```python
from build123d import *

# Parameters (mm, degrees)
BOSS_EXTRUDE1_DEPTH = 10.16
CUT_EXTRUDE1_DEPTH  = 10
CHAMFER1_SIZE       = 0.25
CHAMFER1_SIZE2      = 1.27
SKETCH3_R           = 1.778
BOSS_EXTRUDE2_DEPTH = 0.152
SKETCH4_R           = 0.889
CUT_EXTRUDE2_DEPTH  = 5.08
BOSS_EXTRUDE3_START = 0.9525
BOSS_EXTRUDE3_DEPTH = 0.9525
BOSS_EXTRUDE4_START = 0.318
BOSS_EXTRUDE4_DEPTH = 0.318
BOSS_EXTRUDE5_START = 0.635
SKETCH9_R           = 1.143
BOSS_EXTRUDE5_DEPTH = 0.635
CUT_EXTRUDE3_REACH  = 18.592
SKETCH11_R          = 0.64
CUT_EXTRUDE4_DEPTH  = 6.7
SKETCH12_R          = 0.64
CUT_EXTRUDE6_DEPTH  = 4
CUT_EXTRUDE7_DEPTH  = 1.27
SKETCH15_R          = 0.125
CUT_EXTRUDE8_DEPTH  = 14.860565005


with BuildPart() as part:
    # Sketch1 → Boss-Extrude1 (new, symmetric)
    with BuildSketch(Plane(origin=(0, 0, 0), x_dir=(0, 0, -1), z_dir=(1, 0, 0))):
        Polygon((-9.94, -3.81), (2, -3.81), (2, 3.81), (-7.4, 3.81), (-7.4, 4.57), (-9.18, 4.57), (-9.94, 4.293), align=None)
    extrude(amount=BOSS_EXTRUDE1_DEPTH, both=True)

    # Sketch2 → Cut-Extrude1 (cut)
    with BuildSketch(Plane.XY.offset(9.94)):
        with BuildLine():
            Line((-0.809711007, -2.81), (0.809711007, -2.81))
            ThreePointArc((0.809711007, -2.81), (2.54, -3.3), (4.270288993, -2.81))
            Line((4.270288993, -2.81), (5.08, -2.81))
            Line((5.08, -2.81), (5.08, 2.81))
            Line((5.08, 2.81), (-5.08, 2.81))
            Line((-5.08, 2.81), (-5.08, -2.81))
            Line((-5.08, -2.81), (-4.270288993, -2.81))
            ThreePointArc((-4.270288993, -2.81), (-2.54, -3.3), (-0.809711007, -2.81))
        make_face()
    extrude(amount=-CUT_EXTRUDE1_DEPTH, mode=Mode.SUBTRACT)

    # Chamfer1
    chamfer1_edges = [part.edges().sort_by_distance(p)[0] for p in [
        (-5.08, 0, 9.94),
        (-4.675144497, -2.81, 9.94),
        (-2.54, -3.3, 9.94),
        (0, -2.81, 9.94),
        (2.54, -3.3, 9.94),
        (4.675144497, -2.81, 9.94),
        (5.08, 0, 9.94),
        (0, 2.81, 9.94),
    ]]
    chamfer1_side = [part.faces().sort_by_distance(p)[0] for p in [
        (-9.941239627, 0.2415, 9.94),
    ]]
    chamfer(chamfer1_edges, length=CHAMFER1_SIZE, length2=CHAMFER1_SIZE2, reference=chamfer1_side[0])

    # Sketch3 → Boss-Extrude2 (add)
    with BuildSketch(Plane.XY.offset(9.94)):
        with Locations(Location((-7.62, 0, 0), (0, 0, 180))):
            Circle(SKETCH3_R)
        with Locations(Location((7.76, 0, 0), (0, 0, 180))):
            Circle(SKETCH3_R)
    extrude(amount=BOSS_EXTRUDE2_DEPTH)

    # Sketch4 → Cut-Extrude2 (cut)
    with BuildSketch(Plane.XY.offset(10.092)):
        with Locations((-7.62, 0)):
            Circle(SKETCH4_R)
        with Locations((7.76, 0)):
            Circle(SKETCH4_R)
    extrude(amount=-CUT_EXTRUDE2_DEPTH, mode=Mode.SUBTRACT)

    # Sketch5 → Boss-Extrude3 (add)
    with BuildSketch(Plane.XY.offset(-0.06).offset(BOSS_EXTRUDE3_START)):
        with BuildLine():
            Line((-3.175, 2.81), (-3.175, 1.662881535))
            ThreePointArc((-3.175, 1.662881535), (-3.798650071, 1.258650071), (-4.202881535, 0.635))
            Line((-4.202881535, 0.635), (-5.08, 0.635))
            Line((-5.08, 0.635), (-5.08, -0.635))
            Line((-5.08, -0.635), (-4.202881535, -0.635))
            ThreePointArc((-4.202881535, -0.635), (-3.798650071, -1.258650071), (-3.175, -1.662881535))
            Line((-3.175, -1.662881535), (-3.175, -3.238329044))
            ThreePointArc((-3.175, -3.238329044), (-2.54, -3.3), (-1.905, -3.238329044))
            Line((-1.905, -3.238329044), (-1.905, -1.662881535))
            ThreePointArc((-1.905, -1.662881535), (-1.281349929, -1.258650071), (-0.877118465, -0.635))
            Line((-0.877118465, -0.635), (0, -0.635))
            Line((0, -0.635), (0, 0.635))
            Line((0, 0.635), (-0.877118465, 0.635))
            ThreePointArc((-0.877118465, 0.635), (-1.281349929, 1.258650071), (-1.905, 1.662881535))
            Line((-1.905, 1.662881535), (-1.905, 2.81))
            Line((-1.905, 2.81), (-3.175, 2.81))
        make_face()
    boss_extrude3 = extrude(amount=-BOSS_EXTRUDE3_DEPTH)

    # Mirror1: Boss-Extrude3 across plane
    add(boss_extrude3.mirror(Plane(origin=(0, 0, 0), x_dir=(0, 0, 1), z_dir=(1, 0, 0))))

    # Sketch8 → Boss-Extrude4 (add)
    with BuildSketch(Plane.XY.offset(0.8925).offset(BOSS_EXTRUDE4_START)):
        with BuildLine():
            Line((-4.202881535, 0.635), (-3.490380976, 0.635))
            ThreePointArc((-3.490380976, 0.635), (-2.54, 1.143), (-1.589619024, 0.635))
            Line((-1.589619024, 0.635), (-0.877118465, 0.635))
            Line((-0.877118465, 0.635), (0.877118465, 0.635))
            Line((0.877118465, 0.635), (1.589619024, 0.635))
            ThreePointArc((1.589619024, 0.635), (2.54, 1.143), (3.490380976, 0.635))
            Line((3.490380976, 0.635), (4.202881535, 0.635))
            Line((4.202881535, 0.635), (5.08, 0.635))
            Line((5.08, 0.635), (5.08, -0.635))
            Line((5.08, -0.635), (4.202881535, -0.635))
            ThreePointArc((4.202881535, -0.635), (3.798650071, -1.258650071), (3.175, -1.662881535))
            Line((3.175, -1.662881535), (3.175, -3.238329044))
            ThreePointArc((3.175, -3.238329044), (2.54, -3.3), (1.905, -3.238329044))
            Line((1.905, -3.238329044), (1.905, -1.662881535))
            ThreePointArc((1.905, -1.662881535), (1.281349929, -1.258650071), (0.877118465, -0.635))
            Line((0.877118465, -0.635), (-0.877118465, -0.635))
            ThreePointArc((-0.877118465, -0.635), (-1.281349929, -1.258650071), (-1.905, -1.662881535))
            Line((-1.905, -1.662881535), (-1.905, -3.238329044))
            ThreePointArc((-1.905, -3.238329044), (-2.54, -3.3), (-3.175, -3.238329044))
            Line((-3.175, -3.238329044), (-3.175, -1.662881535))
            ThreePointArc((-3.175, -1.662881535), (-3.798650071, -1.258650071), (-4.202881535, -0.635))
            Line((-4.202881535, -0.635), (-5.08, -0.635))
            Line((-5.08, -0.635), (-5.08, 0.635))
            Line((-5.08, 0.635), (-4.202881535, 0.635))
        make_face()
    extrude(amount=-BOSS_EXTRUDE4_DEPTH)

    # Sketch9 → Boss-Extrude5 (add)
    with BuildSketch(Plane.XY.offset(1.2105).offset(BOSS_EXTRUDE5_START)):
        with Locations(Location((-2.54, 0, 0), (0, 0, 146.251011404))):
            Circle(SKETCH9_R)
        with Locations(Location((2.54, 0, 0), (0, 0, 146.251011404))):
            Circle(SKETCH9_R)
    extrude(amount=-BOSS_EXTRUDE5_DEPTH)

    # Cut-Extrude3: up to this face of the body (flat: up to its plane)
    cut_extrude3_end = Plane(part.part.faces().sort_by_distance((0, 2.81, 4.414046423))[0])
    # Sketch10 → Cut-Extrude3 (cut, up to the picked face)
    with BuildSketch(Plane(origin=(0, 4.57, 0), x_dir=(1, 0, 0), z_dir=(0, 1, 0)), mode=Mode.PRIVATE) as cut_extrude3_sk1:
        Polygon((-2.04, -9.18), (-1.765, -9.94), (-3.315, -9.94), (-3.04, -9.18), align=None)
    cut_extrude3_tool1 = split(extrude(cut_extrude3_sk1.sketch, amount=-CUT_EXTRUDE3_REACH, mode=Mode.PRIVATE), bisect_by=cut_extrude3_end, keep=Keep.BOTH, mode=Mode.PRIVATE)
    # Sketch10 → Cut-Extrude3 (cut, up to the picked face)
    with BuildSketch(Plane(origin=(0, 4.57, 0), x_dir=(1, 0, 0), z_dir=(0, 1, 0)), mode=Mode.PRIVATE) as cut_extrude3_sk2:
        Polygon((-8.395, -9.94), (-8.12, -9.18), (-7.12, -9.18), (-6.845, -9.94), align=None)
    cut_extrude3_tool2 = split(extrude(cut_extrude3_sk2.sketch, amount=-CUT_EXTRUDE3_REACH, mode=Mode.PRIVATE), bisect_by=cut_extrude3_end, keep=Keep.BOTH, mode=Mode.PRIVATE)
    # Sketch10 → Cut-Extrude3 (cut, up to the picked face)
    with BuildSketch(Plane(origin=(0, 4.57, 0), x_dir=(1, 0, 0), z_dir=(0, 1, 0)), mode=Mode.PRIVATE) as cut_extrude3_sk3:
        Polygon((3.04, -9.18), (3.315, -9.94), (1.765, -9.94), (2.04, -9.18), align=None)
    cut_extrude3_tool3 = split(extrude(cut_extrude3_sk3.sketch, amount=-CUT_EXTRUDE3_REACH, mode=Mode.PRIVATE), bisect_by=cut_extrude3_end, keep=Keep.BOTH, mode=Mode.PRIVATE)
    # Sketch10 → Cut-Extrude3 (cut, up to the picked face)
    with BuildSketch(Plane(origin=(0, 4.57, 0), x_dir=(1, 0, 0), z_dir=(0, 1, 0)), mode=Mode.PRIVATE) as cut_extrude3_sk4:
        Polygon((8.12, -9.18), (8.395, -9.94), (6.845, -9.94), (7.12, -9.18), align=None)
    cut_extrude3_tool4 = split(extrude(cut_extrude3_sk4.sketch, amount=-CUT_EXTRUDE3_REACH, mode=Mode.PRIVATE), bisect_by=cut_extrude3_end, keep=Keep.BOTH, mode=Mode.PRIVATE)
    add(cut_extrude3_tool1.solids().sort_by(Axis((-2.54, 4.57, 9.58732), (0, -1, 0)))[0], mode=Mode.SUBTRACT)
    add(cut_extrude3_tool2.solids().sort_by(Axis((-7.62, 4.57, 9.58732), (0, -1, 0)))[0], mode=Mode.SUBTRACT)
    add(cut_extrude3_tool3.solids().sort_by(Axis((2.54, 4.57, 9.58732), (0, -1, 0)))[0], mode=Mode.SUBTRACT)
    add(cut_extrude3_tool4.solids().sort_by(Axis((7.62, 4.57, 9.58732), (0, -1, 0)))[0], mode=Mode.SUBTRACT)

    # Sketch11 → Cut-Extrude4 (cut)
    with BuildSketch(Plane.XZ.offset(3.81)):
        with Locations(Location((-7.62, 2, 0), (0, 0, 270))):
            Circle(SKETCH11_R)
        with Locations(Location((7.62, 2, 0), (0, 0, 270))):
            Circle(SKETCH11_R)
    extrude(amount=-CUT_EXTRUDE4_DEPTH, mode=Mode.SUBTRACT)

    # Sketch12 → Cut-Extrude6 (cut)
    with BuildSketch(Plane(origin=(0, 0, -2), x_dir=(-1, 0, 0), z_dir=(0, 0, -1))):
        with Locations((-7.76, 0)):
            Circle(SKETCH12_R)
        with Locations((7.62, 0)):
            Circle(SKETCH12_R)
    extrude(amount=-CUT_EXTRUDE6_DEPTH, mode=Mode.SUBTRACT)

    # Sketch13 → Cut-Extrude7 (cut, symmetric)
    with BuildSketch(Plane(origin=(2.54, 0, 0), x_dir=(0, 0, -1), z_dir=(1, 0, 0))):
        Polygon((2, -3.81), (2, 2.79), (1.49, 2.79), (1.49, 1.02), (0.73, 1.02), (0.73, -3.56), (-0.92, -3.56), (-1.17, -3.81), align=None)
    cut_extrude7 = extrude(amount=CUT_EXTRUDE7_DEPTH, both=True, mode=Mode.SUBTRACT)

    # Mirror2: Cut-Extrude7 across plane
    add(cut_extrude7.mirror(Plane(origin=(0, 0, 0), x_dir=(0, 0, 1), z_dir=(1, 0, 0))), mode=Mode.SUBTRACT)

    # Sketch15 → Cut-Extrude8 (cut, through all)
    with BuildSketch(Plane.XY.offset(1.8455)):
        with Locations((-2.54, 0)):
            Circle(SKETCH15_R)
        with Locations((2.54, 0)):
            Circle(SKETCH15_R)
    extrude(amount=-CUT_EXTRUDE8_DEPTH, mode=Mode.SUBTRACT)


solid = part.part
```
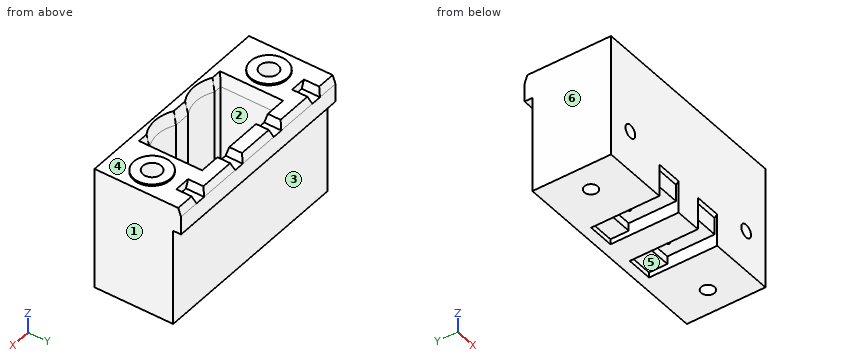
Part model, mm, in its own coordinate system. Face numbers are marked on the shaded views. A direction names the side the tool comes from. Round coordinates to 2 decimals unless told otherwise and drop trailing zeros. Loops run counter-clockwise (first coordinate to the right, second up) from the corner with the lowest first, then second, coordinate; pieces in that order, holes last.
1. Two-plate mould, pull along Y, no slides. Class the marked faces 1, 2 and 3: pulls with the +Y half, pulls with the -Y half, needs draft (parallel to the pull), parting line crosses it, or undercut.
Solutions:
face 1: needs draft
face 2: undercut
face 3: pulls with the +Y half
2. Slice it at D-D (z = 6.5). Give the cut face in (x, y), and give its area (3 significant figures).
Solutions:
outline: (-10.16, -3.81) - (10.16, -3.81) - (10.16, 3.81) - (-10.16, 3.81) - close; hole circle Ø1.78 at (-7.62, 0); hole (-5.08, -2.81) - (-4.27, -2.81) arc R3.3 ccw to (-0.81, -2.81) - (0.81, -2.81) arc R3.3 ccw to (4.27, -2.81) - (5.08, -2.81) - (5.08, 2.81) - (-5.08, 2.81) - close; hole circle Ø1.78 at (7.76, 0)
area: 90.5 mm2
3. 3-axis set-ups, long thin cutter, end or side, ignore diameter. For the marked faces 4, 5 and 6: which of +Z, -Z, +X, -X, +Y, -Y reach the whole face in a straight line?
Solutions:
face 4: +Z
face 5: -Z, -Y
face 6: +Z, -Z, -X, +Y, -Y
4. Slice it at A-A (y = 2.5). Give the cut face in (x, z) (1 decimal).
Solutions:
outline: (-10.2, -2) - (-3.8, -2) - (-3.8, -1.5) - (-1.3, -1.5) - (-1.3, -2) - (1.3, -2) - (1.3, -1.5) - (3.8, -1.5) - (3.8, -2) - (10.2, -2) - (10.2, 9.9) - (5.3, 9.9) - (5.1, 8.7) - (5.1, -0.1) - (3.2, -0.1) - (3.2, 0.9) - (1.9, 0.9) - (1.9, -0.1) - (-1.9, -0.1) - (-1.9, 0.9) - (-3.2, 0.9) - (-3.2, -0.1) - (-5.1, -0.1) - (-5.1, 8.7) - (-5.3, 9.9) - (-10.2, 9.9) - close; hole circle Ø1.3 at (-7.6, 2); hole circle Ø1.3 at (7.6, 2)
5. Slice it at C-C (x = 7.62). Give the cut face in (y, z), and give its area (3 significant figures).
Solutions:
outline: (-3.81, -2) - (-0.62, -2) - (-0.62, 1.36) - (-3.81, 1.36) - close; (-3.81, 2.64) - (2.89, 2.64) - (2.89, 1.36) - (0.62, 1.36) - (0.62, -2) - (3.81, -2) - (3.81, 7.4) - (4.57, 7.4) - (4.57, 9.18) - (2.81, 9.18) - (2.81, 9.94) - (1.77, 9.94) - (1.77, 10.09) - (0.88, 10.09) - (0.88, 5.01) - (-0.88, 5.01) - (-0.88, 10.09) - (-1.77, 10.09) - (-1.77, 9.94) - (-3.81, 9.94) - close
area: 70.4 mm2
6. Drill centre lines: line 1 along X through (y, z) = (-1.25, 1); line 2 along X through (y, z) = (-2.25, 3.5); line 3 along Y through (x, z) = (7.76, 7.85). Where is each one in solid material? Low to high.
Solutions:
line 1: x = -10.16 to -5.08, -3.81 to -1.27, 1.27 to 3.81, 5.08 to 10.16
line 2: x = -10.16 to -5.08, 5.08 to 10.16
line 3: y = -3.81 to -0.89, 0.89 to 4.57
7. Flat gauge pins, fed straight in: pin 1 (1 mm diameter, centred on x = 1.5, y = 2, fed in from +Z); pin 2 (1.4 mm diameter, centred on x = 4.5, z = 0.5, fed in from +Y); pin 3 (1 mm diameter, centred on x = 0.5, y = 3.5, fed in from +Z). Where does each tip first touch, or does it go through?
Solutions:
pin 1: stops at z = 0.89
pin 2: stops at y = 3.81
pin 3: stops at z = 9.94
8. Slice it at B-B (z = -0.5). Give the cut face in (x, y) (3 decimals), and give its area (3 significant figures).
Solutions:
outline: (-10.16, -3.81) - (-3.81, -3.81) - (-3.81, -3.56) - (-1.27, -3.56) - (-1.27, -3.81) - (1.27, -3.81) - (1.27, -3.56) - (3.81, -3.56) - (3.81, -3.81) - (10.16, -3.81) - (10.16, 3.81) - (-10.16, 3.81) - close; hole circle Ø1.28 at (-7.62, 0); hole circle Ø0.25 at (-2.54, 0); hole circle Ø0.25 at (2.54, 0); hole circle Ø1.28 at (7.76, 0)
area: 151 mm2
